from build123d import *

# Parameters (mm, degrees)
SKETCH104_R  = 1.5
PAD053_DEPTH = 4
FILLET082_R  = 4


with BuildPart() as part:
    # Sketch104 → Pad053 (new body)
    with BuildSketch(Plane.XY):
        with BuildLine():
            Line((8.485281, 0), (15, -6.514719))
            Line((15, -39.447222), (15, -6.514719))
            Line((7.424621, -47.022601), (15, -39.447222))
            Line((-47.022601, 7.424621), (7.424621, -47.022601))
            Line((-39.447222, 15), (-47.022601, 7.424621))
            Line((-6.514719, 15), (-39.447222, 15))
            Line((-6.514719, 15), (0, 8.485281))
            Line((0, 8.485281), (-4.242641, 4.242641))
            ThreePointArc((-4.242641, 4.242641), (-4.242641, -4.242641), (4.242641, -4.242641))
            Line((4.242641, -4.242641), (8.485281, 0))
        make_face()
        with Locations((-11.667262, 11.667262)):
            Circle(SKETCH104_R, mode=Mode.SUBTRACT)
        with Locations((-11.667262, -11.667262)):
            Circle(SKETCH104_R, mode=Mode.SUBTRACT)
        with Locations((11.667262, -11.667262)):
            Circle(SKETCH104_R, mode=Mode.SUBTRACT)
    extrude(amount=PAD053_DEPTH)

    # Fillet082
    fillet082_edges = [part.edges().sort_by_distance(p)[0] for p in [
        (7.424621, -47.022601, 2),
        (15, -39.447222, 2),
        (-47.022601, 7.424621, 2),
        (-39.447222, 15, 2),
        (15, -6.514719, 2),
        (-6.514719, 15, 2),
        (8.485281, 0, 2),
        (0, 8.485281, 2),
    ]]
    fillet(fillet082_edges, radius=FILLET082_R)


with BuildPart() as part_1:
    # Body019 placement: moved
    add(part.part.moved(Location((0, 0, 236))))


solid = part_1.part
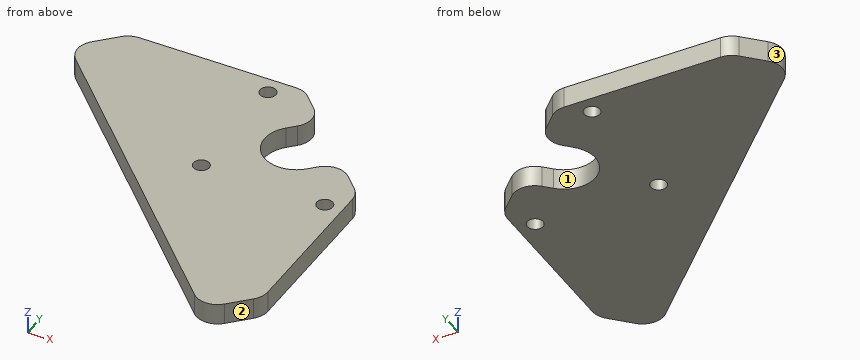
Build history of the part. All positions in model axes, mm. Face numbers are marked on the shaded views. Round coordinates to 2 decimals unless told otherwise and drop trailing zeros. Loops run counter-clockwise (first coordinate to the right, second up) from the corner with the lowest first, then second, coordinate; pieces in that order, holes last. Notation, with made-up numbers: (-26, 89.5) -> (15, 89.5) arc R24 cw to (15, 114.5) -> close; hole circle Ø5 at (-7.5, -11). An arc over 180 degrees is marked (long way). Answer in a Markdown table with one row per item.
Item 1: Saw through at A-A (z = 237.6). Write the cut outline in (x, y), and give its area (3 significant figures).
Answers below:
| item | result |
|---|---|
| outline | (-44.19, 4.6) -> (4.6, -44.19) arc R4 ccw to (10.25, -44.19) -> (13.83, -40.62) arc R4 ccw to (15, -37.79) -> (15, -8.17) arc R4 ccw to (13.83, -5.34) -> (11.31, -2.83) arc R4 ccw to (5.66, -2.83) -> (4.24, -4.24) arc R6 cw to (-4.24, 4.24) -> (-2.83, 5.66) arc R4 ccw to (-2.83, 11.31) -> (-5.34, 13.83) arc R4 ccw to (-8.17, 15) -> (-37.79, 15) arc R4 ccw to (-40.62, 13.83) -> (-44.19, 10.25) arc R4 ccw to start; hole circle Ø3 at (-11.67, -11.67); hole circle Ø3 at (-11.67, 11.67); hole circle Ø3 at (11.67, -11.67) |
| area | 1,910 mm² |
Item 2: Drill centre lines: L1, parallel to Y at x = 12, z = 238.5; L2, parallel to Y at x = -5.5, z = 239; L3, parallel to Y at x = 6, z = 237.55. Where is each one in solid material? Low to high. Write a range as [from, to].
Answers below:
| item | result |
|---|---|
| L1 | y = [-42.45, -13.13], [-10.2, -3.51] |
| L2 | y = [-34.1, -2.4], [2.4, 13.98] |
| L3 | y = [-45.1, -2.52] |
Item 3: Saw through at D-D (x = -21.5). Write the cut outline in (y, z).
Answers below:
| item | result |
|---|---|
| outline | (-18.1, 236) -> (15, 236) -> (15, 240) -> (-18.1, 240) -> close |
Item 4: Saw through at B-B (x = -12). Write the cut outline in (y, z), and give its area (3 significant figures).
Answers below:
| item | result |
|---|---|
| outline | (-27.6, 236) -> (-13.13, 236) -> (-13.13, 240) -> (-27.6, 240) -> close; (-10.2, 236) -> (10.2, 236) -> (10.2, 240) -> (-10.2, 240) -> close; (13.13, 236) -> (15, 236) -> (15, 240) -> (13.13, 240) -> close |
| area | 147 mm² |
Item 5: Saw through at C-C (y = -26). Write the cut outline in (x, z), and give its area (3 significant figures).
Answers below:
| item | result |
|---|---|
| outline | (-13.6, 236) -> (15, 236) -> (15, 240) -> (-13.6, 240) -> close |
| area | 114 mm² |
Item 6: Mould opens along Y. For the marked faces 1, 2 and 3 say: +Y half, -Y half, draft (parallel to the pull), parting line (faces both ways), or undercut.
Answers below:
| item | result |
|---|---|
| face 1 | undercut |
| face 2 | -Y half |
| face 3 | parting line |
Item 7: Pin check, flat tips, straight feed: pin 1 (2.5 mm diameter, centred on x = -11.67, y = -11.67, fed in from -Z); pin 2 (4 mm diameter, centred on x = -11.67, y = 11.67, fed in from +Z); pin 3 (1.5 mm diameter, centred on x = -14.5, z = 239, fed in from -Y). Stop position of each tip, or through.
Answers below:
| item | result |
|---|---|
| pin 1 | passes through |
| pin 2 | stops at z = 240 |
| pin 3 | stops at y = -25.85 |
